Geometry: see drawing. Coordinates: mm, zero at the bounding-box minimum. A direction names the side the tool comes from. Coordinates: 2 decimals unless noted, no trailing zeros. Loops run counter-clockwise (first coordinate to the right, second up) from the corner with the lowest first, then second, coordinate; pieces in that order, holes last.
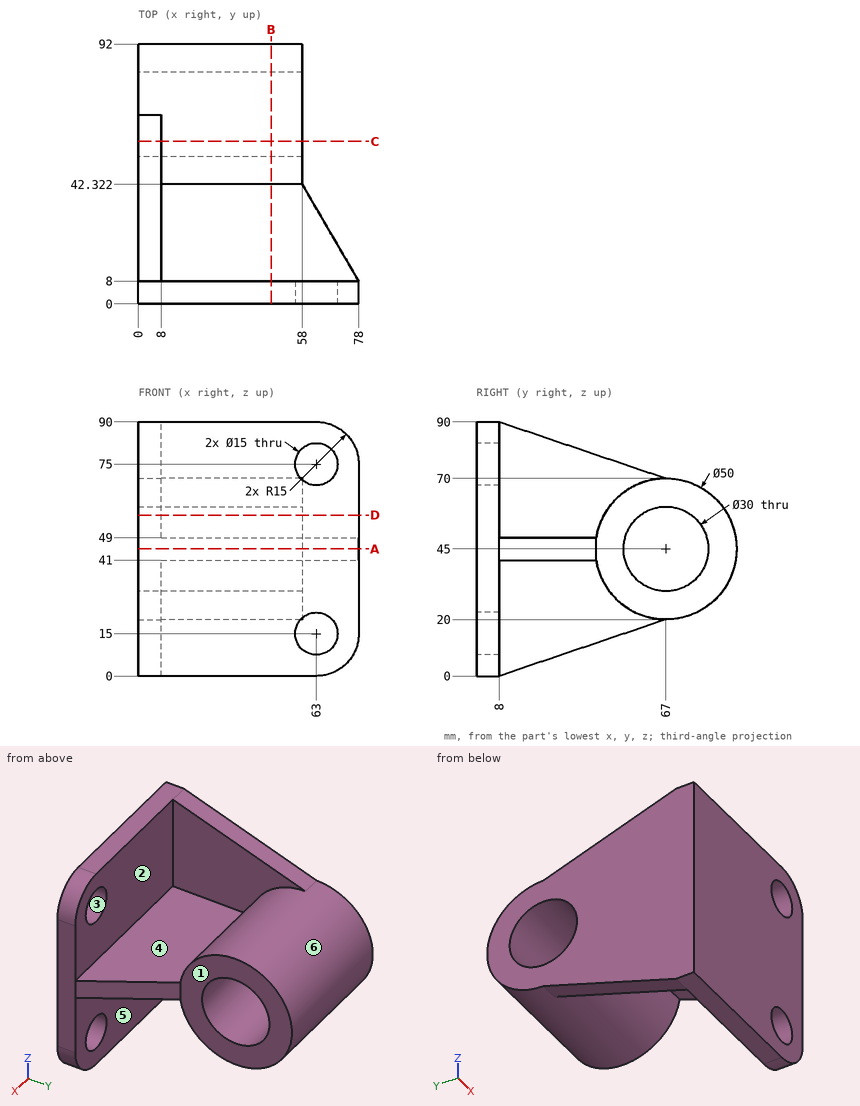
Item 1: Contact query for flat-ended pins moving along their axis: P1, Ø17, axis at x = 58, y = 21.5, coming from the -Z side; P2, Ø2, axis at x = 36, y = 52, coming from the -Z side; P3, Ø4, axis at x = 16, z = 40, coming from the +Y side. Output: stop coordinate, or through.
Result:
P1: stops at z = 41
P2: stops at z = 24.29
P3: stops at y = 91.82
Item 2: Section query D-D (z = 57). Output: boundary loops of the cut face in (x, y), then the cut area to 3 significant figures.
Result:
outline: (0, 0) - (78, 0) - (78, 8) - (8, 8) - (8, 45.07) - (58, 45.07) - (58, 58) - (0, 58) - close; (0, 76) - (58, 76) - (58, 88.93) - (0, 88.93) - close
area: 2,420 mm2
Item 3: Section query B-B (x = 47). Output: boundary loops of the cut face in (y, z), then the cut area to 3 significant figures.
Result:
outline: (0, 0) - (8, 0) - (8, 41) - (42.32, 41) arc R25 ccw (long way) to (42.32, 49) - (8, 49) - (8, 90) - (0, 90) - close; hole circle Ø30 at (67, 45)
area: 2,250 mm2
Item 4: Section query A-A (z = 45). Output: boundary loops of the cut face in (x, y).
Result:
outline: (0, 0) - (78, 0) - (78, 8) - (58, 42.32) - (58, 52) - (0, 52) - close; (0, 82) - (58, 82) - (58, 92) - (0, 92) - close
Item 5: Line query: L1, parallel to Z at x = 63, y = 6; L2, parallel to X at y = 2.75, z = 75; L3, parallel to Y at x = 13, z = 51. Output: solid intervals per line, ascending.
Result:
L1: z = 0 to 7.5, 22.5 to 67.5, 82.5 to 90
L2: x = 0 to 55.5, 70.5 to 78
L3: y = 0 to 8, 42.73 to 53.25, 80.75 to 91.27
Item 6: Section query C-C (y = 57.5). Output: boundary loops of the cut face in (x, z), then the cut area to 3 significant figures.
Result:
outline: (0, 16.78) - (8, 16.78) - (8, 21.88) - (58, 21.88) - (58, 33.39) - (0, 33.39) - close; (0, 56.61) - (58, 56.61) - (58, 68.12) - (8, 68.12) - (8, 73.22) - (0, 73.22) - close
area: 1,420 mm2
Item 7: Reachability of the marked faces 4, 5 and 6 from +Z, -Z, +X, -X, +Y, -Y: full face, straight path, thin tool, end or side. Return the list, or none.
Result:
face 4: +Z, +X
face 5: -Z, +X
face 6: +X
Item 8: Mould query, pull axis X, two halves, no side actions, for the marked faces 1, 2 and 3. Classes: +X half, -X half, draft (parallel to the pull), parting line (faces both ways), or undercut.
Result:
face 1: +X half
face 2: draft
face 3: undercut
